Design review of the part built by this model. Coordinates are the model's own, in mm. Give positions to 0.01 mm unless a question says otherwise; leave off trailing zeros. Write each loop counter-clockwise with the first axis right and the second up, starting at its lowest first coordinate (ties: lowest second). Pieces come first, ordered by that corner, then holes. Notation, with made-up numbers: (70.25, 61.25) - (102.25, 61.25) arc R16 cw to (102.25, 71.25) - close; hole circle Ø5 at (33, -8). An arc over 180 degrees is marked (long way). Write each question's results on one line, items separated by ' | '. Start each with the question number.
from build123d import *

# Parameters (mm, degrees)
CYLINDER002_R           = 40
CYLINDER002_DEPTH       = 100
CYLINDER002_PITCH_ANGLE = 90
CYLINDER001_R           = 15
CYLINDER001_DEPTH       = 736.104612
CYLINDER001_ROLL_ANGLE  = -10


with BuildPart() as eje_brazo:
    # Cylinder002 → Cylinder002 (new body)
    with BuildSketch(Plane.XY):
        Circle(CYLINDER002_R)
    extrude(amount=CYLINDER002_DEPTH)


with BuildPart() as eje_brazo_1:
    # Cylinder002 pitch: moved
    add(eje_brazo.part.rotate(Axis((0, 0, 0), (0, 1, 0)), CYLINDER002_PITCH_ANGLE))


with BuildPart() as eje_brazo_2:
    # Cylinder002 placement: moved
    add(eje_brazo_1.part.moved(Location((-59, 715, 400))))


with BuildPart() as brazo:
    # Cylinder001 → Cylinder001 (new body)
    with BuildSketch(Plane.XY):
        Circle(CYLINDER001_R)
    extrude(amount=CYLINDER001_DEPTH)


with BuildPart() as brazo_1:
    # Cylinder001 roll: moved
    add(brazo.part.rotate(Axis((0, 0, 0), (1, 0, 0)), CYLINDER001_ROLL_ANGLE))


with BuildPart() as brazo_2:
    # Cylinder001 placement: moved
    add(brazo_1.part.moved(Location((-40, 715, 400))))

    # Fusion: union Eje_brazo
    add(eje_brazo_2.part)


with BuildPart() as obj1:
    # mirror: instance of Brazo
    add(brazo_2.part.mirror(Plane(origin=(500, 0, 0), x_dir=(0, -1, 0), z_dir=(1, 0, 0))))


solid = obj1.part
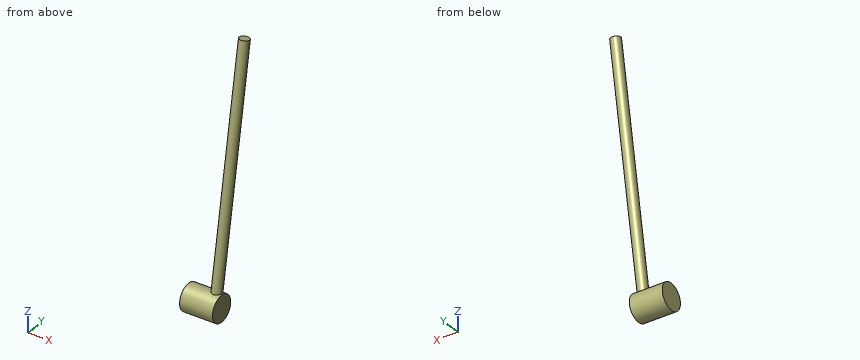
Q1. Insertion check: P1, Ø5, axis at x = 975, y = 724, coming from the +Z side; P2, Ø12, axis at y = 817, z = 1043, coming from the -X side; P3, Ø6, axis at x = 1000.5, y = 718, coming from the +Z side. Each pin has a flat end and moves straight along its axis. Give the tip position at first contact, or say it passes through.
Q2. For line 1 along Y through (x, z) = (1037.5, 403.5); line 2 along Y through (x, z) = (1036, 829); line 3 along Z through (x, y) = (1002, 688.5), list the stretches that pass through material, from the lowest coordinate up. Write a range as [from, to].
Q3. Add section C-C on y = 689. State the section outline as (x, z) points, plus the area to 3 significant figures.
Q4. Add section B-B on z = 400. State the section outline as (x, y) points.
Q5. Add section A-A on x = 1011. State the section outline as (y, z) points, plus the area to 3 significant figures.
Result:
1) P1: stops at z = 439.47 | P2: stops at x = 1025.93 | P3: stops at z = 440
2) line 1: y = [675.15, 754.85] | line 2: y = [775.96, 805.32] | line 3: z = [370.04, 429.96]
3) outline: (959, 369.6) - (1059, 369.6) - (1059, 430.4) - (959, 430.4) - close | area: 6,080 mm²
4) outline: (959, 675) - (1059, 675) - (1059, 755) - (959, 755) - close
5) outline: circle Ø80 at (715, 400) | area: 5,030 mm²
